Solid Edge part; units mm, degrees
sketch "Sketch1" plane through (0, 0, 0) normal (0, -1, 0) x (1, 0, 0)
  line L0 (0, 0) -> (0, -24)
  line L1 (0, -24) -> (40, -24)
  line L2 (40, -24) -> (40, 0)
  line L3 (40, 0) -> (0, 0)
extrude "Protrusion1" add sketch "Sketch1" along normal blind 10
sketch "Sketch2" plane through (20, -10, -12) normal (0, -1, 0) x (1, 0, 0)
  circle A0 centre (-1.5, 0) radius 3.2
extrude "ExtrudedCutout_1" cut sketch "Sketch2" against normal blind 73.4208
sketch "Sketch3" plane through (20, -5, -12) normal (0, 0, -1) x (-1, 0, 0)
  line L0 (0, 5) -> (14.5, 5)
  line L1 (14.5, 5) -> (17, -1.4)
  line L2 (17, -1.4) -> (0, -1.4)
revolve "RevolvedCutout1" cut sketch "Sketch3" angle 360 about axis through (20, -10, -12) along (0, -1, 0)
sketch "Sketch4" plane through (20, -5, -12) normal (0, 0, -1) x (-1, 0, 0)
  line L0 (-20, 5) -> (-33.5002, 5)
  line L1 (-33.5002, 5) -> (-33.5002, -5)
  line L2 (-33.5002, -5) -> (-20, -5)
  line L3 (-20, -5) -> (-20, 5)
  line L4 (20, 5) -> (20, -5)
  line L5 (20, -5) -> (28, -5)
  line L6 (28, -5) -> (28, 5)
  line L7 (28, 5) -> (20, 5)
  dimension "D1" = 28
extrude "Protrusion2" add sketch "Sketch4" along normal up to surface (24 mm away) from surface at -12
sketch "Sketch5" plane through (22.7501, -5, 0) normal (0, 0, 1) x (-1, 0, 0)
  spline S0 degree 3 poles (-5.3893, -5) (-6.1043, -3.9725) (-6.7754, -2.9183) (-8.0674, -0.7797) (-8.6877, 0.3051) (-9.2915, 1.4) knots 0 0 0 0 0.5 0.5 1 1 1 1
  line L0 (-9.2915, 1.4) -> (-4.8846, 1.4)
  line L1 (-4.8846, 1.4) -> (10.7035, 1.4)
  line L2 (10.7035, 1.4) -> (14.7917, 1.4)
  line L3 (14.7917, 1.4) -> (10.8895, -5)
  line L4 (10.8895, -5) -> (30.7501, -5)
  line L5 (30.7501, -5) -> (30.7501, 5)
  line L6 (30.7501, 5) -> (-30.7501, 5)
  line L7 (-30.7501, 5) -> (-30.7501, -5)
  line L8 (-5.3893, -5) -> (-30.7501, -5)
extrude "Protrusion3" add sketch "Sketch5" along normal up to vertex (2 mm away)
sketch "Sketch6" plane through (22.7501, -5, 2) normal (0, 0, 1) x (-1, 0, 0)
  line L0 (32.2203, -5) -> (30.7501, -5)
  line L1 (30.7501, 5) -> (30.7501, -5)
  line L2 (32.2203, 5) -> (30.7501, 5)
  line L3 (32.2203, -5) -> (32.2203, 5)
extrude "Protrusion4" add sketch "Sketch6" against normal up to vertex (26 mm away)
sketch "Sketch7" plane through (22.015, -10, -11) normal (0, -1, 0) x (-1, 0, 0)
  line L0 (-28.4852, 3.2) -> (-20.4852, 3.2)
  line L1 (-20.4852, 3.2) -> (-20.4852, -1.2)
  line L2 (-20.4852, -1.2) -> (-28.4852, -1.2)
  line L3 (-28.4852, -1.2) -> (-28.4852, 3.2)
  dimension "D1" = 28.4852
  dimension "D2" = 20.4852
extrude "ExtrudedCutout_3" cut sketch "Sketch7" against normal blind 37.6385
mirror "Mirror1" about plane through (22.0152, -5, -11) normal (1, 0, 0) of "ExtrudedCutout_3"
sketch "Sketch8" plane through (22.015, -10, -11) normal (0, -1, 0) x (-1, 0, 0)
  line L0 (-1.485, 4.2) -> (-1.485, -2.2007)
  line L1 (-1.485, -2.2007) -> (8.515, -2.2007)
  line L2 (8.515, -2.2007) -> (8.515, 4.2)
  line L3 (8.515, 4.2) -> (-1.485, 4.2)
  dimension "D1" = 1.485
  dimension "D2" = 8.515
extrude "ExtrudedCutout_4" cut sketch "Sketch8" against normal blind 87.6344
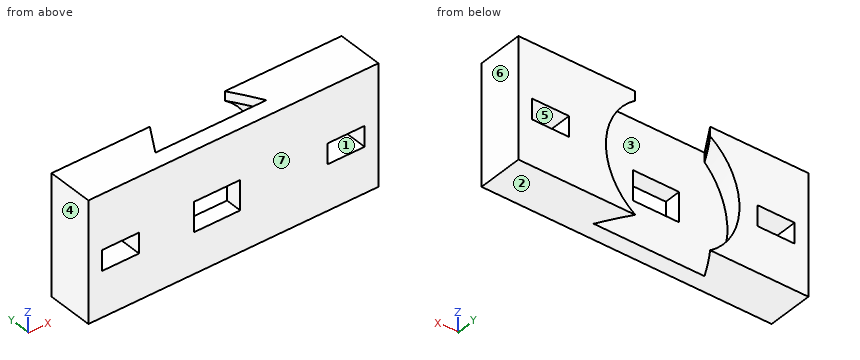
Verification items for the finished model (mm, model axes). Face numbers are marked on the shaded views. A direction names the side the tool comes from. Give positions to 0.01 mm unless a question says otherwise; leave off trailing zeros. Loops run counter-clockwise (first coordinate to the right, second up) from the corner with the lowest first, then second, coordinate; pieces in that order, holes last.
1. Mould release check, pull along X, two halves, no side actions. Record for the marked faces 4, 5, 6 and 7: released by +X, released by -X, zero draft, split by the parting line, or undercut.
2. Section check C-C, the plane x = 17. Enter the section's corners in (y, z).
3. Set-up check for the marked faces 1, 2 and 3: record each of +Z, -Z, +X, -X, +Y, -Y from which the full face is reachable in a straight line by a thin tool's end or side.
4. Section check B-B, the plane y = -7. Enter the section's corners in (x, z).
5. Go/stop test with a flat-tipped pin: pin 1 Ø8 at (x, z) = (24, -7.5) entering from +Y. Record where the tip stops, or that it passes through.
6. Section check D-D, the plane z = -11. Count the separate pieces of the cut face and the enclosed holes in it, then the cut area to 3 significant figures.
7. Section check A-A, the plane x = 46. Enter the section's corners in (y, z), then the cut area to 3 significant figures.
8. Thickness scan on line 1 (X direction, y = -7.5, z = -12); line 2 (Z direction, x = -6, y = -7); line 3 (X direction, y = -2.25, z = 1.25). Record the ranges inside material, lowest first.
Geometry says:
1. face 4: released by -X
1. face 5: undercut
1. face 6: released by +X
1. face 7: zero draft
2. outline: (-10, -24) - (-6.4, -24) - (-6.4, -15.2) - (-10, -15.2) - close; (-10, -8.8) - (-6.4, -8.8) - (-6.4, 2) - (-10, 2) - close
3. face 1: +Y, -Y
3. face 2: -Z, +X, -X, +Y, -Y
3. face 3: none
4. outline: (-9.47, -24) - (53.5, -24) - (53.5, 2) - (-9.47, 2) - close; hole (-6.47, -14.2) - (1.53, -14.2) - (1.53, -9.8) - (-6.47, -9.8) - close; hole (13.5, -15.2) - (23.5, -15.2) - (23.5, -8.8) - (13.5, -8.8) - close; hole (42.5, -14.2) - (50.5, -14.2) - (50.5, -9.8) - (42.5, -9.8) - close
5. pin 1: stops at y = -6.4
6. separate pieces: 4
6. enclosed holes: 0
6. area: 233 mm2
7. outline: (-10, -24) - (0, -24) - (0, -14.2) - (-10, -14.2) - close; (-10, -9.8) - (0, -9.8) - (0, 2) - (-10, 2) - close
7. area: 216 mm2
8. line 1: x = -9.47 to -6.47, 1.53 to 13.5, 23.5 to 42.5, 50.5 to 53.5
8. line 2: z = -24 to -14.2, -9.8 to 2
8. line 3: x = -9.47 to 10.49, 29.62 to 53.5
